Check sheet for the drawn part. Datum: minimum x, y, z corner. Units: mm. Give positions to 0.01 mm unless a question says otherwise; leave off trailing zeros. Order: outer loops, then holes, each group sorted by start corner. A loop starts at its lowest first (then second) coordinate and runs counter-clockwise, first axis right, second up. Notation, with made-up numbers: (-25, -26.5) -> (27, -26.5) arc R21 ccw to (27, -19.5) -> close; hole circle Ø8 at (52.25, 5). An arc over 180 degrees is marked (long way). One line per question, with ' | ' between items. Start each with the question number.
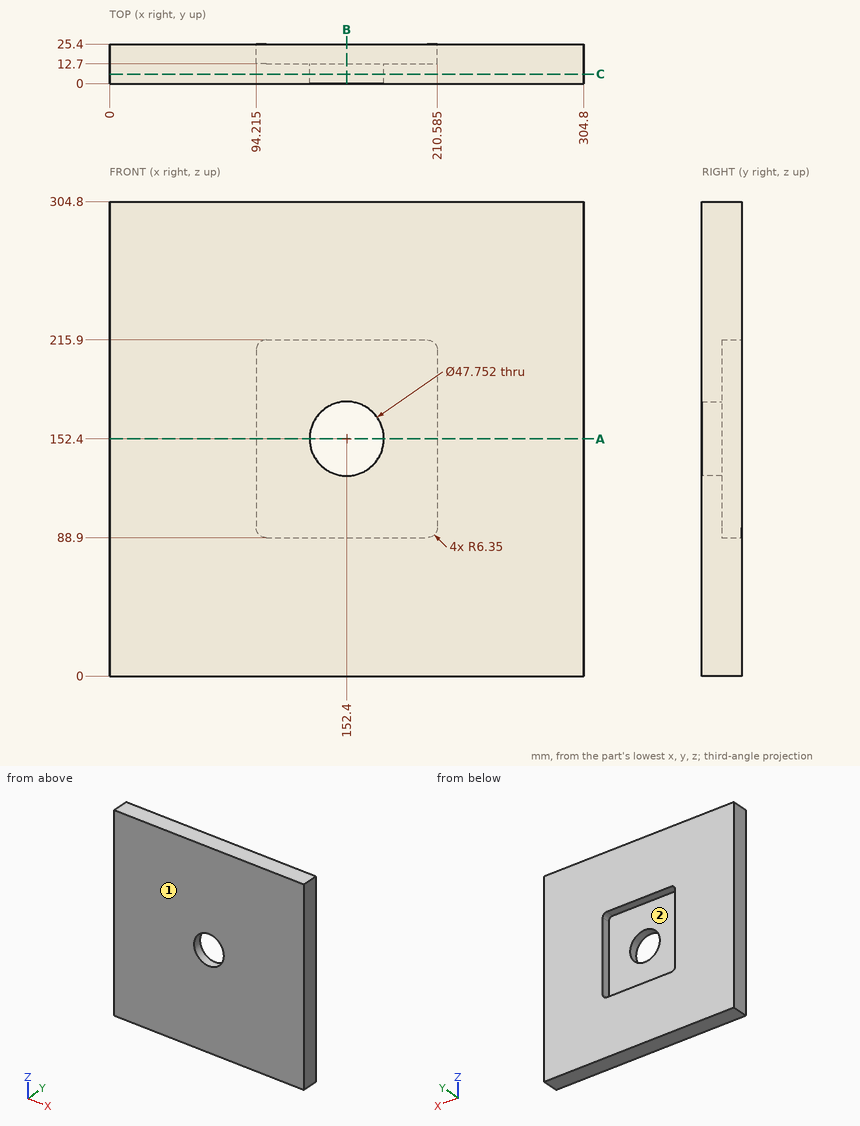
1. Cross-section at B-B on x = 152.4. Record the boundary of the cut face in (y, z), and give its area (3 significant figures).
2. Scan lines: probe 1 along X at (y, z) = (4, 152.4); probe 2 along Z at (x, y) = (107.5, 18.75); probe 3 along X at (y, z) = (19.75, 90.5). Record each from-to range of solid material in increasing order.
3. Mould release check, pull along X, two halves, no side actions. Record for the marked faces 1 and 2: +X half, -X half, draft (parallel to the pull), parting line (faces both ways), or undercut.
4. Cross-section at A-A on z = 152.4. Record the boundary of the cut face in (x, y) (1 decimal), and give its area (3 significant figures).
5. Cross-section at C-C on y = 6. Record the boundary of the cut face in (x, z).
Response values:
1) outline: (0, 0) -> (25.4, 0) -> (25.4, 88.9) -> (12.7, 88.9) -> (12.7, 128.52) -> (0, 128.52) -> close; (0, 176.28) -> (12.7, 176.28) -> (12.7, 215.9) -> (25.4, 215.9) -> (25.4, 304.8) -> (0, 304.8) -> close | area: 5,520 mm²
2) probe 1: x = 0 to 128.52, 176.28 to 304.8 | probe 2: z = 0 to 88.9, 215.9 to 304.8 | probe 3: x = 0 to 96.35, 208.45 to 304.8
3) face 1: draft | face 2: undercut
4) outline: (0, 0) -> (128.5, 0) -> (128.5, 12.7) -> (94.2, 12.7) -> (94.2, 25.4) -> (0, 25.4) -> close; (176.3, 0) -> (304.8, 0) -> (304.8, 25.4) -> (210.6, 25.4) -> (210.6, 12.7) -> (176.3, 12.7) -> close | area: 5,660 mm²
5) outline: (0, 0) -> (304.8, 0) -> (304.8, 304.8) -> (0, 304.8) -> close; hole circle Ø47.75 at (152.4, 152.4)
